Drawing for the job (mm, zero at the part's lowest x, y, z). A direction names the side the tool comes from. Round coordinates to 2 decimals unless told otherwise and drop trailing zeros. Order: outer loops, then holes, each group sorted by start corner. A loop starts at its lowest first (then second) coordinate and runs counter-clockwise, first axis right, second up. Notation, with made-up numbers: (21, -6.75) -> (69, -6.75) arc R24 ccw to (69, 10.25) -> close; hole circle Ø4 at (-33.5, 79.5). An arc over 180 degrees is marked (long way). Use CSV: the item, a comma, the result in double quotes.
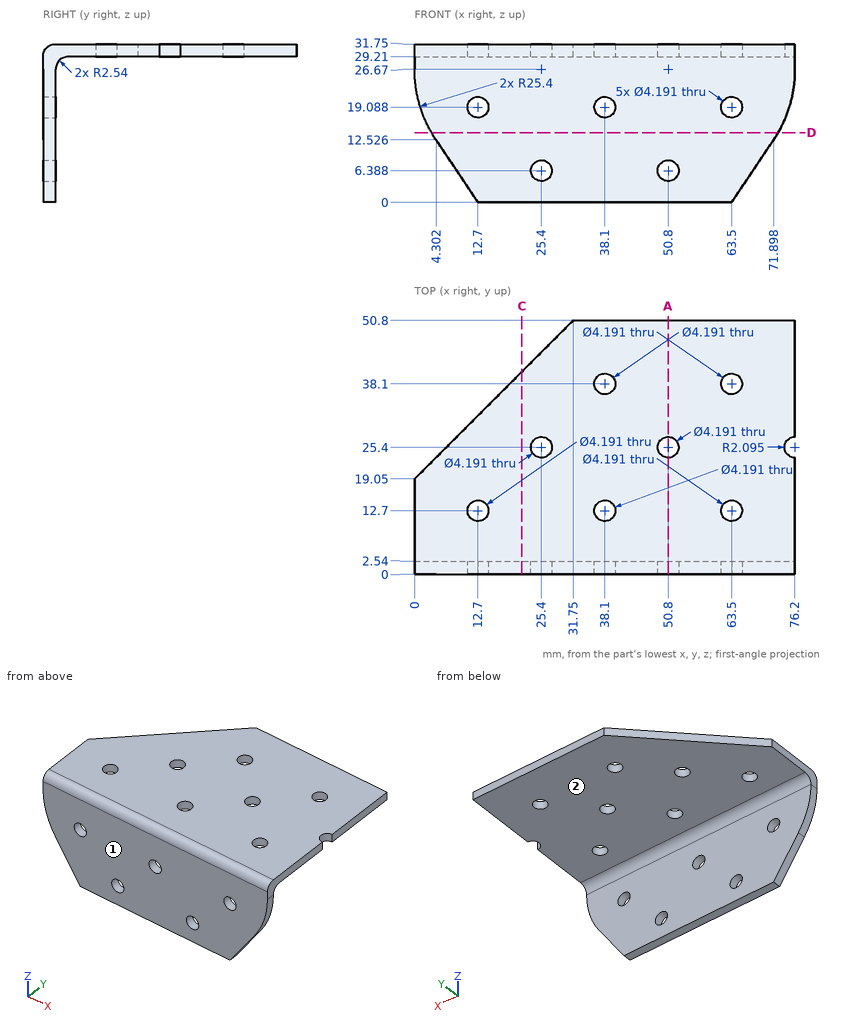
Q1. Cut at C-C (x = 21.5). Give the cut face in (y, z), plus the area to 3 significant figures.
From the geometry:
outline,"(0, 0) -> (2.54, 0) -> (2.54, 26.67) arc R2.54 cw to (5.08, 29.21) -> (40.55, 29.21) -> (40.55, 31.75) -> (2.54, 31.75) arc R2.54 ccw to (0, 29.21) -> close"
area,"177 mm²"
Q2. Probe line 1 along Y through (x, z) = (38.1, 30.8) (1 decimal); line 2 along Z through (x, y) = (25, 36.5); line 3 along Y through (x, z) = (67.5, 8). List the from-to ranges inside material, lowest first.
From the geometry:
line 1,"y = 0.6 to 10.6, 14.8 to 36, 40.2 to 50.8"
line 2,"z = 29.21 to 31.75"
line 3,"y = 0 to 2.54"
Q3. Pin check, flat tips, straight feed: pin 1 (3.5 mm diameter, centred on x = 38.1, z = 19.09, fed in from +Y); pin 2 (5 mm diameter, centred on x = 63.5, z = 19.09, fed in from +Y); pin 3 (5 mm diameter, centred on x = 46, y = 17.5, fed in from -Z). Stop position of each tip, or through.
From the geometry:
pin 1,"passes through"
pin 2,"stops at y = 2.54"
pin 3,"stops at z = 29.21"
Q4. Cut at A-A (x = 50.8). State how many separate pieces and enclosed holes the cut face has, plus the area to 3 significant figures.
From the geometry:
separate pieces,"3"
enclosed holes,"0"
area,"182 mm²"
Q5. Cut at D-D (z = 14). Give the cut face in (x, y) (1 decimal), plus the area to 3 significant figures.
From the geometry:
outline,"(3.4, 0) -> (72.8, 0) -> (72.8, 2.5) -> (3.4, 2.5) -> close"
area,"176 mm²"
Q6. Which spindle directions (+Z, -Z, +X, -X, +Y, -Y) get a long thin tool onto all of the face, cutting with end or side? Do the marked faces 1 and 2. Say none if no direction does.
From the geometry:
face 1,"+Z, -Z, +X, -X, -Y"
face 2,"-Z, +X, -X, +Y"
